Geometry check sheet. Reference: the model listing, model coordinates, mm. A direction names the side the tool comes from. Give positions to 0.01 mm unless a question says otherwise; leave off trailing zeros. Write each loop counter-clockwise with the first axis right and the second up, starting at its lowest first coordinate (ties: lowest second). Pieces come first, ordered by that corner, then holes.
(1) Mould release check, pull along Y, two halves, no side actions. Record for faces 4 (the flat face through (-13, -32.5, 2)), 5 (the flat face through (-22.5, -28, 2)), 6 (the flat face through (-14.1, -19, 3)), 7 (the flat face through (15, 32.5, 2)): +Y half, -Y half, draft (parallel to the pull), parting line (faces both ways), or undercut.
(2) Cross-section at B-B (y = -21.5). Record the boundary of the cut face in (x, z), and give its area (3 significant figures).
(3) Cross-section at A-A (x = -16.5). Record the boundary of the cut face in (y, z).
(4) Depth check by flat-ended pin: P1, Ø1, axis at x = -15, z = 1.5, coming from the +Y side; P2, Ø2, axis at y = -22, z = 3.5, coming from the +X side; P3, Ø1.3, axis at y = -21.5, z = 2.5, coming from the -X side. Enter the tip coordinate at first touch or a pass-through.
(5) Thickness scan on line 1 along Y through (x, z) = (18.5, 1.4); line 2 along Y through (x, z) = (0, 2.8); line 3 along Y through (x, z) = (-20, 3.55). Record the ranges inside material, lowest first.
(6) Tool access check on faces 1 (the flat face through (14.1, 25, 3)), 2 (the flat face through (-11, -20.1, 3)), 3 (the flat face through (11, -20.1, 3)). Record the directions out of +Z, -Z, +X, -X, +Y, -Y that give a thin tool (end or side, any length) a straight path to the whole face; none if there is none.
```python
from build123d import *

# Parameters (mm, degrees)
BOSS_EXTRUDE1_DEPTH = 5
CUT_EXTRUDE1_DEPTH  = 5
SKETCH5_R           = 4
SKETCH5_R_2         = 2
BOSS_EXTRUDE2_DEPTH = 5
SKETCH6_R           = 2
CUT_EXTRUDE2_DEPTH  = 5


with BuildPart() as part:
    # Sketch1 → Boss-Extrude1 (new body)
    with BuildSketch(Plane.XY):
        Polygon((7.5, 32.5), (7.5, 37.5), (-7.5, 37.5), (-7.5, 32.5), (-22.5, 32.5), (-22.5, -32.5), (22.5, -32.5), (22.5, 32.5), align=None)
    extrude(amount=BOSS_EXTRUDE1_DEPTH)

    # Sketch3 → Cut-Extrude1 (cut)
    with BuildSketch(Plane.XY.offset(5)):
        Polygon((22.5, 24.5), (17.5, 24.5), (17.5, 26), (14.1, 26), (14.1, 24.5), (7.5, 24.5), (7.5, 20.1), (14.1, 20.1), (14.1, 18.6), (17.5, 18.6), (17.5, 20.1), (22.5, 20.1), align=None)
        Polygon((22.5, -24.5), (22.5, -20.1), (17.5, -20.1), (17.5, -18.6), (14.1, -18.6), (14.1, -20.1), (7.5, -20.1), (7.5, -24.5), (14.1, -24.5), (14.1, -26), (17.5, -26), (17.5, -24.5), align=None)
        Polygon((-22.5, -24.5), (-17.5, -24.5), (-17.5, -26), (-14.1, -26), (-14.1, -24.5), (-7.5, -24.5), (-7.5, -20.1), (-14.1, -20.1), (-14.1, -18.6), (-17.5, -18.6), (-17.5, -20.1), (-22.5, -20.1), align=None)
    extrude(amount=-CUT_EXTRUDE1_DEPTH, mode=Mode.SUBTRACT)

    # Sketch5 → Boss-Extrude2 (add)
    with BuildSketch(Plane.XY.offset(5)):
        with Locations((0, -32.5)):
            Circle(SKETCH5_R)
        with Locations((0, -32.5)):
            Circle(SKETCH5_R_2, mode=Mode.SUBTRACT)
    extrude(amount=-BOSS_EXTRUDE2_DEPTH)

    # Sketch6 → Cut-Extrude2 (cut)
    with BuildSketch(Plane.XY.offset(5)):
        with Locations((0, -32.5)):
            Circle(SKETCH6_R)
    extrude(amount=-CUT_EXTRUDE2_DEPTH, mode=Mode.SUBTRACT)


solid = part.part
```
Reply:
1. face 4: -Y half
1. face 5: draft
1. face 6: undercut
1. face 7: +Y half
2. outline: (-7.5, 0) - (7.5, 0) - (7.5, 5) - (-7.5, 5) - close
2. area: 75.0 mm2
3. outline: (-32.5, 0) - (-26, 0) - (-26, 5) - (-32.5, 5) - close; (-18.6, 0) - (32.5, 0) - (32.5, 5) - (-18.6, 5) - close
4. P1: stops at y = 32.5
4. P2: stops at x = 7.5
4. P3: stops at x = -7.5
5. line 1: y = -32.5 to -24.5, -20.1 to 20.1, 24.5 to 32.5
5. line 2: y = -36.5 to -34.5, -30.5 to 37.5
5. line 3: y = -32.5 to -24.5, -20.1 to 32.5
6. face 1: +Z, -Z
6. face 2: +Z, -Z, -X
6. face 3: +Z, -Z, +X
